Geometry check sheet. Reference: drawing and pictorial views, mm from the part's lowest x, y, z. Round coordinates to 2 decimals unless told otherwise and drop trailing zeros. Write each loop counter-clockwise with the first axis right and the second up, starting at its lowest first coordinate (ties: lowest second). Pieces come first, ordered by that corner, then holes. Notation, with made-up numbers: M -11.5,-3 L -3.5,-3 A10 cw -3.5,15 Z; hole C -0.5,13.25 d8. An arc over 180 degrees is marked long. One line per question, with ' | ' between items.
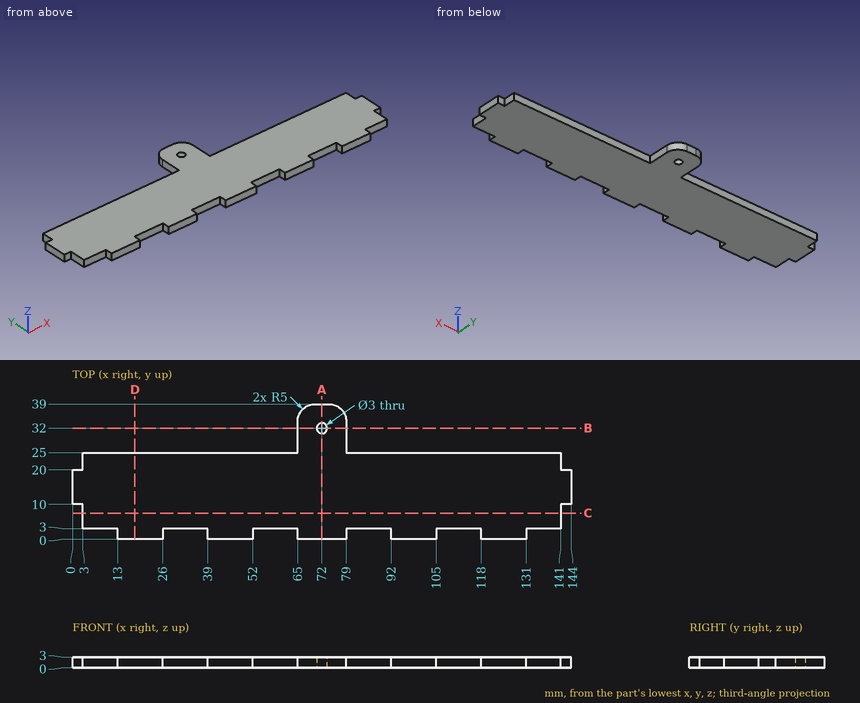
1. Section check C-C, the plane y = 7.5. Record the cut outline in (x, z), then the cut area to 3 significant figures.
Results:
outline: M 3,0 L 141,0 L 141,3 L 3,3 Z | area: 414 mm2
2. Section check B-B, the plane y = 32. Record the cut outline in (x, z).
Results:
outline: M 65,0 L 70.5,0 L 70.5,3 L 65,3 Z; M 73.5,0 L 79,0 L 79,3 L 73.5,3 Z
3. Section check D-D, the plane x = 18. Record the cut outline in (y, z).
Results:
outline: M 0,0 L 25,0 L 25,3 L 0,3 Z
4. Go/stop test with flat-tipped pins: P1, Ø1.5, axis at y = 22.5, z = 1.5, coming from the -X side; P2, Ø0.9, axis at y = 30.5, z = 1, coming from the +X side; P3, Ø1.5, axis at x = 27.5, z = 1.5, coming from the +Y side. Record where each tip stops, or that it passes through.
Results:
P1: stops at x = 3 | P2: stops at x = 79 | P3: stops at y = 25
5. Thickness scan on line 1 (Y direction, x = 72, z = 0.75); line 2 (X direction, y = 2.5, z = 1.95); line 3 (X direction, y = 23.5, z = 0.45). Record the ranges inside material, lowest first.
Results:
line 1: y = 0 to 30.5, 33.5 to 39 | line 2: x = 13 to 26, 39 to 52, 65 to 79, 92 to 105, 118 to 131 | line 3: x = 3 to 141
6. Section check A-A, the plane x = 72. Record the cut outline in (y, z).
Results:
outline: M 0,0 L 30.5,0 L 30.5,3 L 0,3 Z; M 33.5,0 L 39,0 L 39,3 L 33.5,3 Z
